Design review of the part built by this model. Coordinates are the model's own, in mm. Face numbers are marked on the shaded views. Give positions to 0.01 mm unless a question says otherwise; leave off trailing zeros. Write each loop counter-clockwise with the first axis right and the second up, starting at its lowest first coordinate (ties: lowest second). Pieces come first, ordered by that corner, then holes. Notation, with made-up numbers: M 56.25,6.5 L 100.25,6.5 A32 ccw 100.25,45.5 Z; hole C 79,11 d1. An arc over 180 degrees is marked long. One line per item, written item: value. Start each with the question number.
```python
from build123d import *

# Parameters (mm, degrees)
SKETCH1_R          = 16.75
SKETCH2_R          = 21
SKETCH1_4_R        = 2.75
SKETCH1_4_R_2      = 10
CUT_EXTRUDE1_DEPTH = 8.5000001


with BuildPart() as part:
    # Sketch1 → Loft1 section 0
    with BuildSketch(Plane(origin=(0, 0, 0), x_dir=(1, 0, 0), z_dir=(0, 1, 0))):
        Circle(SKETCH1_R)
    # Sketch2 → Loft1 section 1
    with BuildSketch(Plane(origin=(0, 7.5, 0), x_dir=(1, 0, 0), z_dir=(0, 1, 0))):
        Circle(SKETCH2_R)
    loft()

    # Sketch1<4> → Cut-Extrude1 (cut, through all)
    with BuildSketch(Plane(origin=(0, 0, 0), x_dir=(1, 0, 0), z_dir=(0, 1, 0))):
        with Locations((-16.694272111, 1.365202803)):
            Circle(SKETCH1_4_R)
        with Locations((-9.529436364, -13.775062344)):
            Circle(SKETCH1_4_R)
        with Locations((9.529436364, 13.775062344)):
            Circle(SKETCH1_4_R)
        with Locations((-7.164835747, 15.140265147)):
            Circle(SKETCH1_4_R)
        Circle(SKETCH1_4_R_2)
        with Locations((7.164835747, -15.140265147)):
            Circle(SKETCH1_4_R)
        with Locations((16.694272111, -1.365202803)):
            Circle(SKETCH1_4_R)
    extrude(amount=CUT_EXTRUDE1_DEPTH, mode=Mode.SUBTRACT)


solid = part.part
```
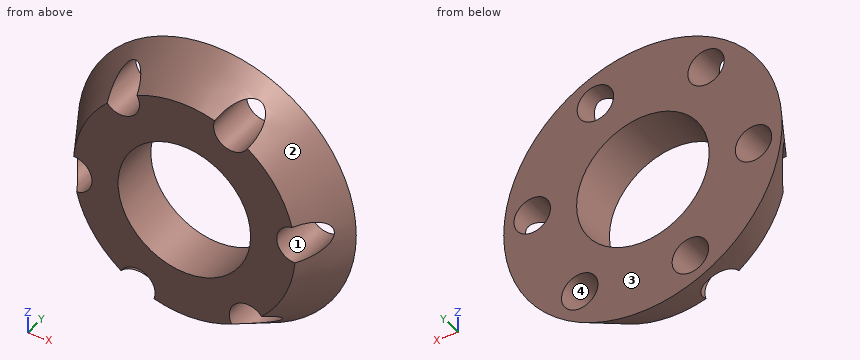
Q1. Take a section at C-C, the plane z = 0. State how many separate pieces and enclosed holes the cut face has, then the cut area to 3 significant figures.
Q2. Take a section at B-B, the plane y = 5.5. Give the boundary of the cut face in (x, z).
Q3. Take a section at A-A, the plane x = 0. Give the boundary of the cut face in (y, z).
Q4. Wall thickness on line 1 (X direction, y = 6.75, z = 13); line 2 (X direction, y = 6.25, z = 12); line 3 (Z direction, x = -1, y = 1.5): over which ranges is each line inside the solid? List them lowest first. Write a range as from..to.
Q5. For P1, Ø2, axis at x = -1.5, y = 4, coming from the -Z side; P2, Ø1, axis at y = 6, z = -1, coming from the +X side; P3, Ø3, axis at x = -7.5, y = 6, coming from the +Z side, all flat-tipped, find the tip position at first contact; note any pin that passes through.
Q6. The part is to be moulded in two halves that separate along Z. For the marked faces 1, 2, 3 and 4, say which applies: pulls with the +Z half, pulls with the -Z half, needs draft (parallel to the pull), parting line crosses it, or undercut.
Results list:
1. separate pieces: 4
1. enclosed holes: 0
1. area: 71.1 mm^2
2. outline: C 0,0 d39.73; hole C -16.69,-1.37 d5.5; hole C -9.53,13.78 d5.5; hole C 0,0 d20; hole C -7.16,-15.14 d5.5; hole C 7.16,15.14 d5.5; hole C 9.53,-13.78 d5.5; hole C 16.69,1.37 d5.5
3. outline: M 0,-16.75 L 7.5,-21 L 7.5,-10 L 0,-10 Z; M 0,10 L 7.5,10 L 7.5,21 L 0,16.75 Z
4. line 1: x = -15.95..-12.17, -6.89..5.44, 8.89..15.95
4. line 2: x = -16.36..-11.63, -7.43..16.36
4. line 3: z = -17.57..-9.95, 9.95..17.57
5. P1: stops at z = -19.53
5. P2: stops at x = 20.41
5. P3: stops at z = 19.77
6. face 1: undercut
6. face 2: parting line crosses it
6. face 3: needs draft
6. face 4: undercut
